```python
from build123d import *


with BuildPart() as part:
    # Schizzo1 → Rivoluzione1 (revolve)
    with BuildSketch(Plane.XZ):
        with BuildLine():
            Line((10.8, 0), (10.8, 10))
            ThreePointArc((10.8, 10), (9.921320344, 12.121320344), (7.8, 13))
            Line((7.8, 13), (1, 13))
            Line((1, 13), (1, 12.75))
            Line((1, 12.75), (7.8, 12.75))
            ThreePointArc((7.8, 12.75), (9.744543648, 11.944543648), (10.55, 10))
            Line((10.55, 10), (10.55, 0))
            Line((10.55, 0), (10.8, 0))
        make_face()
    revolve(axis=Axis((0, 0, 13), (0, 0, -1)))


solid = part.part
```
Source: CAD feature listing. Evaluate the final solid. Frame: model axes, mm. Round coordinates to 2 decimals unless told otherwise and drop trailing zeros. Loops run counter-clockwise (first coordinate to the right, second up) from the corner with the lowest first, then second, coordinate; pieces in that order, holes last. Notation, with made-up numbers: M -19,40.25 L 23,40.25 A34 ccw 23,78.25 Z; hole C -23,78.25 d6. An arc over 180 degrees is marked long. Use a Markdown table: item, result. Add a question column.
1. Contact query for flat-ended pins moving along their axis: P1, Ø1.5, axis at x = 8, z = 2.5, coming from the +Y side; P2, Ø1, axis at x = -7, y = -6.5, coming from the -Z side; P3, Ø2, axis at x = 3.5, y = 5.5, coming from the -Z side. Output: stop coordinate, or through.
2. Section query D-D on z = 12.25. Return the cut outline in (x, y).
3. Section query A-A on y = 0. Return the cut outline in (x, z).
4. Section query C-C on z = 2.5. Return the cut outline in (x, y), then the cut area to 3 significant figures.
5. Line query: line 1 (Y direction, x = 0, z = 4.25); line 2 (Z direction, x = 3.75, y = 4.25); line 3 (Y direction, x = 4, z = 10). Output: solid intervals per line, ascending.
6. Mould query, pull axis Y, two halves, no side actions, for faces 1 (the flat face through (0, 2, 13)), 2 (the cylindrical face through (-2.341, 10.543, 5.07)), 3 (the cylindrical face through (10.063, -3.169, 4.93)). Classes: pulls with the +Y half, pulls with the -Y half, needs draft (parallel to the pull), parting line crosses it, or undercut.
Reported:
| question | item | result |
|---|---|---|
| 1 | P1 | stops at y = 8 |
| 1 | P2 | stops at z = 11.58 |
| 1 | P3 | stops at z = 12.75 |
| 2 | outline | C 0,0 d19.57; hole C 0,0 d18.76 |
| 3 | outline | M -10.8,0 L -10.55,0 L -10.55,10 A2.75 cw -7.8,12.75 L -1,12.75 L -1,13 L -7.8,13 A3 ccw -10.8,10 Z; M 1,12.75 L 7.8,12.75 A2.75 cw 10.55,10 L 10.55,0 L 10.8,0 L 10.8,10 A3 ccw 7.8,13 L 1,13 Z |
| 4 | outline | C 0,0 d21.6; hole C 0,0 d21.1 |
| 4 | area | 16.8 mm² |
| 5 | line 1 | y = -10.8 to -10.55, 10.55 to 10.8 |
| 5 | line 2 | z = 12.75 to 13 |
| 5 | line 3 | y = -10.03 to -9.76, 9.76 to 10.03 |
| 6 | face 1 | needs draft |
| 6 | face 2 | parting line crosses it |
| 6 | face 3 | undercut |
